```python
from build123d import *

# Parameters (mm, degrees)
BOSS_EXTRUDE1_DEPTH                            = 19.05
SKETCH2_W                                      = 63.5
SKETCH2_H                                      = 6.35
CUT_EXTRUDE1_DEPTH                             = 441.730714978
BOSS_EXTRUDE3_DEPTH                            = 19.05
FILLET1_R                                      = 4.7625
CSK_FOR_8_FLAT_HEAD_MACHINE_SCREW1_D           = 4.4958
CSK_FOR_8_FLAT_HEAD_MACHINE_SCREW1_DEPTH       = 30.1752
CSK_FOR_8_FLAT_HEAD_MACHINE_SCREW1_CSINK_D     = 8.4328
CSK_FOR_8_FLAT_HEAD_MACHINE_SCREW1_CSINK_ANGLE = 82
CSK_FOR_8_FLAT_HEAD_MACHINE_SCREW1_TIP         = 1.350674586


with BuildPart() as part:
    # Sketch1 → Boss-Extrude1 (new body)
    with BuildSketch(Plane.XY):
        with BuildLine():
            Line((276.225, 0), (276.225, 330.2))
            ThreePointArc((276.225, 330.2), (272.505256121, 339.180256121), (263.525, 342.9))
            Line((263.525, 342.9), (-263.525, 342.9))
            ThreePointArc((-263.525, 342.9), (-272.505256121, 339.180256121), (-276.225, 330.2))
            Line((-276.225, 330.2), (-276.225, 0))
            Line((-276.225, 0), (-257.175, 0))
            Line((-257.175, 0), (-257.175, 76.2))
            Line((-257.175, 76.2), (-257.175, 165.1))
            ThreePointArc((-257.175, 165.1), (-210.678201513, 277.353201513), (-98.425, 323.85))
            Line((-98.425, 323.85), (98.425, 323.85))
            ThreePointArc((98.425, 323.85), (210.678201513, 277.353201513), (257.175, 165.1))
            Line((257.175, 165.1), (257.175, 76.2))
            Line((257.175, 76.2), (257.175, 0))
            Line((257.175, 0), (276.225, 0))
        make_face()
        with BuildLine():
            Line((250.825, 323.85), (201.795510785, 323.85))
            ThreePointArc((201.795510785, 323.85), (195.725385382, 319.364424197), (198.231010413, 312.244827586))
            ThreePointArc((198.231010413, 312.244827586), (224.148585695, 290.823585695), (245.569827586, 264.906010413))
            ThreePointArc((245.569827586, 264.906010413), (252.689424197, 262.400385382), (257.175, 268.470510785))
            Line((257.175, 268.470510785), (257.175, 317.5))
            ThreePointArc((257.175, 317.5), (255.315128061, 321.990128061), (250.825, 323.85))
        make_face(mode=Mode.SUBTRACT)
        with BuildLine():
            Line((-250.825, 323.85), (-201.795510785, 323.85))
            ThreePointArc((-201.795510785, 323.85), (-195.725385382, 319.364424197), (-198.231010413, 312.244827586))
            ThreePointArc((-198.231010413, 312.244827586), (-224.148585695, 290.823585695), (-245.569827586, 264.906010413))
            ThreePointArc((-245.569827586, 264.906010413), (-252.689424197, 262.400385382), (-257.175, 268.470510785))
            Line((-257.175, 268.470510785), (-257.175, 317.5))
            ThreePointArc((-257.175, 317.5), (-255.315128061, 321.990128061), (-250.825, 323.85))
        make_face(mode=Mode.SUBTRACT)
    extrude(amount=BOSS_EXTRUDE1_DEPTH)

    # Sketch2 → Cut-Extrude1 (cut, through all)
    with BuildSketch(Plane(origin=(0, 342.9, 0), x_dir=(1, 0, 0), z_dir=(0, 1, 0))):
        with Locations((-23.8125, -15.875)):
            Rectangle(SKETCH2_W, SKETCH2_H)
    extrude(amount=-CUT_EXTRUDE1_DEPTH, mode=Mode.SUBTRACT)

    # Sketch3 → Boss-Extrude3 (add)
    with BuildSketch(Plane.XY):
        with BuildLine():
            ThreePointArc((-116.873274525, 322.774422996), (-73.976886998, 309.253399344), (-55.5625, 268.21892))
            Line((-55.5625, 268.21892), (7.9375, 268.21892))
            ThreePointArc((7.9375, 268.21892), (24.231466087, 307.556033913), (63.56858, 323.85))
            Line((63.56858, 323.85), (7.9375, 323.85))
            Line((7.9375, 323.85), (-55.5625, 323.85))
            Line((-55.5625, 323.85), (-98.425, 323.85))
            ThreePointArc((-98.425, 323.85), (-107.664801119, 323.580877633), (-116.873274525, 322.774422996))
        make_face()
    extrude(amount=BOSS_EXTRUDE3_DEPTH)

    # Fillet1
    fillet1_edges = [part.edges().sort_by_distance(p)[0] for p in [
        (-55.5625, 268.21892, 9.525),
        (7.9375, 268.21892, 9.525),
    ]]
    fillet(fillet1_edges, radius=FILLET1_R)

    # CSK for #8 Flat Head Machine Screw1
    with Locations(Plane(origin=(0, 0, 0), x_dir=(-1, 0, 0), z_dir=(0, 0, -1))):
        with Locations((23.813611707, 293.61892), (266.7, 19.05), (-266.7, 19.05)):
            CounterSinkHole(CSK_FOR_8_FLAT_HEAD_MACHINE_SCREW1_D / 2, CSK_FOR_8_FLAT_HEAD_MACHINE_SCREW1_CSINK_D / 2, depth=CSK_FOR_8_FLAT_HEAD_MACHINE_SCREW1_DEPTH, counter_sink_angle=CSK_FOR_8_FLAT_HEAD_MACHINE_SCREW1_CSINK_ANGLE)
            with Locations((0, 0, -(CSK_FOR_8_FLAT_HEAD_MACHINE_SCREW1_DEPTH + CSK_FOR_8_FLAT_HEAD_MACHINE_SCREW1_TIP / 2))):  # 118° drill point
                Cone(0, CSK_FOR_8_FLAT_HEAD_MACHINE_SCREW1_D / 2, CSK_FOR_8_FLAT_HEAD_MACHINE_SCREW1_TIP, mode=Mode.SUBTRACT)


solid = part.part
```
Source: CAD feature listing. Evaluate the final solid. Frame: model axes, mm. A direction names the side the tool comes from. Give positions to 0.01 mm unless a question says otherwise; leave off trailing zeros. Write each loop counter-clockwise with the first axis right and the second up, starting at its lowest first coordinate (ties: lowest second). Pieces come first, ordered by that corner, then holes.
1. Section query D-D (x = -70). Return the cut outline in (y, z).
2. Section query B-B (x = 219.5). Return the cut outline in (y, z).
3. First-contact query: pin 1 (8 mm diameter, centred on x = 4.5, z = 15, fed in from -Y); pin 2 (5.5 mm diameter, centred on x = 86.5, z = 7.5, fed in from -Y); pin 3 (1.9 mm diameter, centred on x = -21.5, z = 15, fed in from +Y). Flat tips, straight axial feed; report the tip coordinate or a pass-through.
4. Access query for faces 1 (the face through (-218.09, 269.417, 9.392)), 2 (the face through (-257.175, 293, 9)), 3 (the face through (-24, 334, 12.7)), 4 (the face through (-1, 274, 0)). Directions: +Z, -Z, +X, -X, +Y, -Y. A direction counts if a zero-diameter tool reaches every point of the face in a straight line with its end or side. Return the directions, or none.
5. Section query A-A (y = 86.5). Return the cut outline in (x, z) (3 decimals).
6. Pull-direction query (Y, two-part tool) for faces 5 (the face through (-267, 0, 9)), 6 (the face through (252.581, 262.368, 9.392)), 7 (the face through (-22, 274, 19.05)), 8 (the face through (-227, 323.85, 9)); classes: +Y half, -Y half, draft (parallel to the pull), parting line (faces both ways), or undercut.
7. Material intervals for line 1 along X through (y, z) = (101, 15) (3 decimals); line 2 along X through (y, z) = (19.05, 13) (3 decimals); line 3 along Y through (x, z) = (70.5, 10), sorted ascending.
8. Section query C-C (z = 5.5). Count the separate pieces of the cut face and the enclosed holes in it, then the cut area to 3 significant figures.
Output values:
1. outline: (305.33, 0) - (342.9, 0) - (342.9, 19.05) - (305.33, 19.05) - close
2. outline: (267.78, 0) - (295.31, 0) - (295.31, 19.05) - (267.78, 19.05) - close; (323.85, 0) - (342.9, 0) - (342.9, 19.05) - (323.85, 19.05) - close
3. pin 1: stops at y = 268.22
3. pin 2: stops at y = 323.85
3. pin 3: stops at y = 323.85
4. face 1: +Z, -Z, -Y
4. face 2: +Z, -Z
4. face 3: +Z, +Y
4. face 4: -Z, +X, -X, +Y, -Y
5. outline: (-276.225, 0) - (-257.175, 0) - (-257.175, 19.05) - (-276.225, 19.05) - close; (257.175, 0) - (276.225, 0) - (276.225, 19.05) - (257.175, 19.05) - close
6. face 5: -Y half
6. face 6: undercut
6. face 7: draft
6. face 8: undercut
7. line 1: x = -276.225 to -257.175, 257.175 to 276.225
7. line 2: x = -276.225 to -268.948, -264.452 to -257.175, 257.175 to 264.452, 268.948 to 276.225
7. line 3: y = 323.85 to 342.9
8. separate pieces: 1
8. enclosed holes: 5
8. area: 34,000 mm2
